```python
from build123d import *

# Parameters (mm, degrees)
SKETCH1_W            = 40
SKETCH1_H            = 40
BOSS_EXTRUDE1_DEPTH  = 2
EXTRUDE_THIN1_START  = 2
SKETCH1_3_W          = 14
SKETCH1_3_H          = 1
EXTRUDE_THIN1_DEPTH  = 11.2
SKETCH3_R            = 1.5
CUT_EXTRUDE1_DEPTH   = 13.2
LPATTERN1_COUNT      = 2
LPATTERN1_PITCH      = 32
LPATTERN1_COUNT_DIR2 = 2
LPATTERN1_PITCH_DIR2 = 32


with BuildPart() as part:
    # Sketch1 → Boss-Extrude1 (new body)
    with BuildSketch(Plane.XY):
        with Locations((21, 22.483732861)):
            Rectangle(SKETCH1_W, SKETCH1_H)
    extrude(amount=BOSS_EXTRUDE1_DEPTH)

    # Sketch1<3> → Extrude-Thin1 (add)
    with BuildSketch(Plane.XY.offset(EXTRUDE_THIN1_START)):
        with Locations((34, 11.415311808)):
            Rectangle(SKETCH1_3_W, SKETCH1_3_H)
        with Locations((34, 14.131101282)):
            Rectangle(SKETCH1_3_W, SKETCH1_3_H)
        with Locations((34, 17.752153914)):
            Rectangle(SKETCH1_3_W, SKETCH1_3_H)
        with Locations((34, 20.467943387)):
            Rectangle(SKETCH1_3_W, SKETCH1_3_H)
        with Locations((34, 23.183732861)):
            Rectangle(SKETCH1_3_W, SKETCH1_3_H)
        with Locations((34, 25.899522335)):
            Rectangle(SKETCH1_3_W, SKETCH1_3_H)
        with Locations((34, 29.520574966)):
            Rectangle(SKETCH1_3_W, SKETCH1_3_H)
        with Locations((34, 32.23636444)):
            Rectangle(SKETCH1_3_W, SKETCH1_3_H)
        with Locations((8, 11.415311808)):
            Rectangle(SKETCH1_3_W, SKETCH1_3_H)
        with Locations((8, 14.131101282)):
            Rectangle(SKETCH1_3_W, SKETCH1_3_H)
        with Locations((8, 17.752153914)):
            Rectangle(SKETCH1_3_W, SKETCH1_3_H)
        with Locations((8, 20.467943387)):
            Rectangle(SKETCH1_3_W, SKETCH1_3_H)
        with Locations((8, 23.183732861)):
            Rectangle(SKETCH1_3_W, SKETCH1_3_H)
        with Locations((8, 25.899522335)):
            Rectangle(SKETCH1_3_W, SKETCH1_3_H)
        with Locations((8, 29.520574966)):
            Rectangle(SKETCH1_3_W, SKETCH1_3_H)
        with Locations((8, 32.23636444)):
            Rectangle(SKETCH1_3_W, SKETCH1_3_H)
    extrude(amount=EXTRUDE_THIN1_DEPTH)

    # Sketch3 → Cut-Extrude1 (cut)
    with BuildSketch(Plane(origin=(0, 0, 0), x_dir=(-1, 0, 0), z_dir=(0, 0, -1))):
        with Locations((-37, 6.483732861)):
            Circle(SKETCH3_R)
    cut_extrude1 = extrude(amount=-CUT_EXTRUDE1_DEPTH, mode=Mode.SUBTRACT)

    # LPattern1: Cut-Extrude1 2 × 2
    with Locations(*[(-i * LPATTERN1_PITCH, j * LPATTERN1_PITCH_DIR2, 0) for i in range(LPATTERN1_COUNT) for j in range(LPATTERN1_COUNT_DIR2) if (i, j) != (0, 0)]):
        add(cut_extrude1, mode=Mode.SUBTRACT)


solid = part.part
```
Geometry check sheet. Reference: the model listing, model coordinates, mm. A direction names the side the tool comes from. Coordinates: 2 decimals unless noted, no trailing zeros. Order: outer loops, then holes, each group sorted by start corner. A loop starts at its lowest first (then second) coordinate and runs counter-clockwise, first axis right, second up.
Item 1: Depth check by flat-ended pin: pin 1 (2 mm diameter, centred on x = 32, z = 10, fed in from -Y); pin 2 (1 mm diameter, centred on x = 30, z = 5.5, fed in from +Y); pin 3 (10 mm diameter, centred on x = 20.5, y = 8, fed in from +Z); pin 4 (1.5 mm diameter, centred on x = 16.5, z = 4.5, fed in from -Y). Enter the tip coordinate at first touch or a pass-through.
Item 2: Section check A-A (y = 6). Enter the section's corners in (x, z), plus the area to 3 significant figures.
Item 3: Mould release check, pull along Y, two halves, no side actions. Record for faces 1 (the cylindrical face through (38.19, 37.57, 0.99)), 2 (the flat face through (27, 20.5, 7.5)), 3 (the flat face through (21, 2.484, 1)): released by +Y, released by -Y, zero draft, split by the parting line, or undercut.
Item 4: Section check B-B (z = 10.25). Count the separate pieces of the cut face and the enclosed holes in it, plus the area to 3 significant figures.
Item 5: Scan lines: line 1 along Y through (x, z) = (5, 0.55); line 2 along X through (y, z) = (32.5, 7.5); line 3 along Z through (x, y) = (28.5, 36). Record each from-to range of solid material in increasing order.
Item 6: Section check D-D (x = 17.5). Enter the section's corners in (y, z).
Item 7: Tool access check on faces 4 (the flat face through (8, 30.021, 8)), 5 (the cylindrical face through (38.19, 5.57, 0.99)), 6 (the flat face through (27, 29.5, 7.5)). Record the directions out of +Z, -Z, +X, -X, +Y, -Y that give a thin tool (end or side, any length) a straight path to the whole face; none if there is none.
Check sheet entries:
1. pin 1: stops at y = 10.92
1. pin 2: stops at y = 32.74
1. pin 3: stops at z = 2
1. pin 4: passes through
2. outline: (1, 0) - (3.58, 0) - (3.58, 2) - (1, 2) - close; (6.42, 0) - (35.58, 0) - (35.58, 2) - (6.42, 2) - close; (38.42, 0) - (41, 0) - (41, 2) - (38.42, 2) - close
2. area: 68.6 mm2
3. face 1: undercut
3. face 2: zero draft
3. face 3: released by -Y
4. separate pieces: 16
4. enclosed holes: 0
4. area: 224 mm2
5. line 1: y = 2.48 to 4.98, 7.98 to 36.98, 39.98 to 42.48
5. line 2: x = 1 to 15, 27 to 41
5. line 3: z = 0 to 2
6. outline: (2.48, 0) - (42.48, 0) - (42.48, 2) - (2.48, 2) - close
7. face 4: +Z, +X, -X
7. face 5: +Z, -Z
7. face 6: +Z, +Y, -Y
